Could you check a few things on this drawing? It's one solid part, dimensions in mm from its lowest x, y, z. Give positions to 0.01 mm unless a question says otherwise; leave off trailing zeros. Order: outer loops, then holes, each group sorted by start corner. A loop starts at its lowest first (then second) coordinate and runs counter-clockwise, first axis right, second up. Notation, with made-up numbers: (79.25, -37) - (136.25, -37) arc R19 cw to (136.25, 0) - close; hole circle Ø11 at (-20.75, 61). An arc over 180 degrees is marked (long way). Put each result on its own line as item: value.
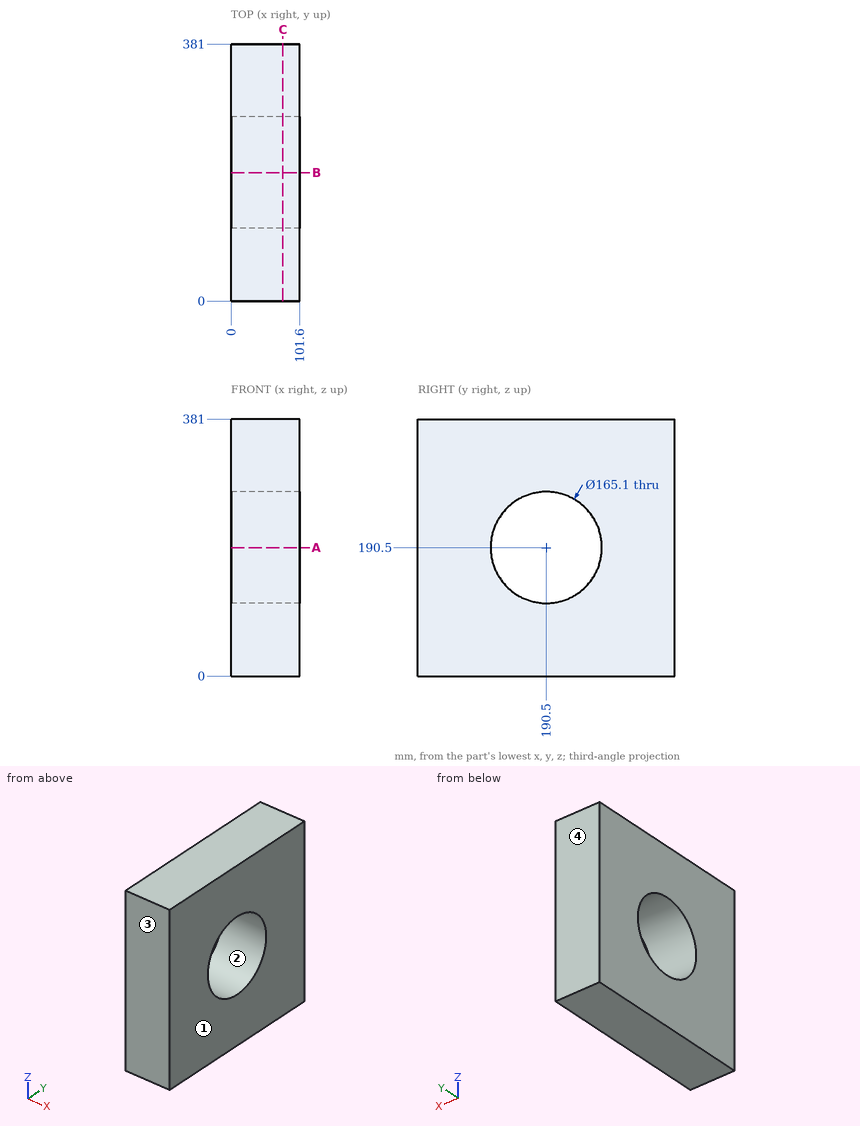
1) I'm going to push a flat-ended pin straight in: pin 1 (4 mm diameter, centred on x = 78, y = 151.5, fed in from -Z). Where does the tip first touch, or does it pass through?
Filled in:
pin 1: stops at z = 0
2) Suppose I cut it at A-A, the plane z = 190.5. List the corners of the cut face in (x, y) for me, and give its area (3 significant figures).
Filled in:
outline: (0, 0) - (101.6, 0) - (101.6, 107.95) - (0, 107.95) - close; (0, 273.05) - (101.6, 273.05) - (101.6, 381) - (0, 381) - close
area: 21,900 mm^2
3) If I drill on line 1 (Y direction, x = 56, z = 190); line 2 (Z direction, x = 79, y = 234.5), over which ranges is the centre line in solid material (lowest first)? Write a range as [from, to].
Filled in:
line 1: y = [0, 107.95], [273.05, 381]
line 2: z = [0, 120.65], [260.35, 381]
4) We'd pull the mould along Y, two halves only. Please class the marked faces 1, 2, 3 and 4: pulls with the +Y half, pulls with the -Y half, needs draft (parallel to the pull), parting line crosses it, or undercut.
Filled in:
face 1: needs draft
face 2: undercut
face 3: pulls with the -Y half
face 4: pulls with the +Y half
5) Suppose I cut it at C-C, the plane x = 76.5. List the corners of the cut face in (y, z) for me, and give its area (3 significant figures).
Filled in:
outline: (0, 0) - (381, 0) - (381, 381) - (0, 381) - close; hole circle Ø165.1 at (190.5, 190.5)
area: 124,000 mm^2
